from build123d import *

# Parameters (mm, degrees)
SKETCH4_W           = 40
SKETCH4_H           = 85
BOSS_EXTRUDE1_DEPTH = 2.5
SKETCH5_W           = 9.5
SKETCH5_H           = 5
BOSS_EXTRUDE2_DEPTH = 2.5
SKETCH12_W          = 9
SKETCH12_H          = 13
CUT_EXTRUDE1_DEPTH  = 5
FILLET4_R           = 1
FILLET5_R           = 1
SKETCH13_R          = 0.75
CUT_EXTRUDE2_DEPTH  = 10


with BuildPart() as part:
    # Sketch4 → Boss-Extrude1 (new body)
    with BuildSketch(Plane(origin=(0, 0, 0), x_dir=(1, 0, 0), z_dir=(0, 1, 0))):
        Rectangle(SKETCH4_W, SKETCH4_H)
    extrude(amount=BOSS_EXTRUDE1_DEPTH)

    # Sketch5 → Boss-Extrude2 (add)
    with BuildSketch(Plane(origin=(0, 2.5, 0), x_dir=(1, 0, 0), z_dir=(0, 1, 0))):
        with Locations((15.25, -45)):
            Rectangle(SKETCH5_W, SKETCH5_H)
    extrude(amount=-BOSS_EXTRUDE2_DEPTH)

    # Sketch12 → Cut-Extrude1 (cut)
    with BuildSketch(Plane(origin=(0, 2.5, 0), x_dir=(1, 0, 0), z_dir=(0, 1, 0))):
        with Locations((-12.75, 31)):
            Rectangle(SKETCH12_W, SKETCH12_H)
    extrude(amount=-CUT_EXTRUDE1_DEPTH, mode=Mode.SUBTRACT)

    # Fillet4
    fillet4_edges = [part.edges().sort_by_distance(p)[0] for p in [
        (15.25, 2.5, 47.5),
    ]]
    fillet(fillet4_edges, radius=FILLET4_R)

    # Fillet5
    fillet5_edges = [part.edges().sort_by_distance(p)[0] for p in [
        (15.25, 0, 47.5),
    ]]
    fillet(fillet5_edges, radius=FILLET5_R)

    # Sketch13 → Cut-Extrude2 (cut)
    with BuildSketch(Plane.ZY.offset(-10.5)):
        with Locations((46.35, 1.25)):
            Circle(SKETCH13_R)
    extrude(amount=-CUT_EXTRUDE2_DEPTH, mode=Mode.SUBTRACT)


solid = part.part
Could you check a few things on this model? Use its own coordinates, in mm. A direction names the side the tool comes from. Coordinates: 2 decimals unless noted, no trailing zeros. Order: outer loops, then holes, each group sorted by start corner. A loop starts at its lowest first (then second) coordinate and runs counter-clockwise, first axis right, second up.
Q1. Which directions (+Z, -Z, +X, -X, +Y, -Y) give clear straight access to the entire face, cutting with the end or side of a thin tool? Please do faces 1 (the flat face through (-20, 1, 1)), 2 (the flat face through (-13, 1, -37.5)), 3 (the flat face through (-5, 1, 42.5)).
Q2. Will these pins go through, and if not, where does the flat tip stop? pin 1 (0.8 mm diameter, centred on y = 1, z = 46, fed in from -X); pin 2 (0.9 mm diameter, centred on y = 1.25, z = 46.35, fed in from +X); pin 3 (1.2 mm diameter, centred on x = -0.5, y = 1, fed in from +Z).
Q3. Please list where these lines run through material, in increasing order: L1, parallel to Z at x = -14, y = 0.15; L2, parallel to Y at x = 18, z = 46.35; L3, parallel to Z at x = -7, y = 2.
Q4. Thinking about a two-plate mould opening in Z: for faces 4 (the flat face through (0, 1, -42.5)), 5 (the flat face through (-17.25, 1, -31)), 6 (the flat face through (0, 2.5, 1)), 7 (the flat face through (-8.25, 1, -31)), which applies, released by +Z, released by -Z, zero draft, split by the parting line, or undercut?
Q5. Suppose I cut it at A-A on x = -11. Please give me the cut outline in (y, z), and give its area (3 significant figures).
Q6. Suppose I cut it at B-B on x = 1. Please give me the cut outline in (y, z), and give its area (4 significant figures).
Answer:
1. face 1: +Z, -Z, -X, +Y, -Y
1. face 2: +Y, -Y
1. face 3: +Z, -X, +Y, -Y
2. pin 1: stops at x = 10.5
2. pin 2: passes through
2. pin 3: stops at z = 42.5
3. L1: z = -42.5 to -37.5, -24.5 to 42.5
3. L2: y = 0 to 0.5, 2 to 2.5
3. L3: z = -42.5 to 42.5
4. face 4: released by -Z
4. face 5: undercut
4. face 6: zero draft
4. face 7: undercut
5. outline: (0, -42.5) - (2.5, -42.5) - (2.5, -37.5) - (0, -37.5) - close; (0, -24.5) - (2.5, -24.5) - (2.5, 42.5) - (0, 42.5) - close
5. area: 180 mm2
6. outline: (0, -42.5) - (2.5, -42.5) - (2.5, 42.5) - (0, 42.5) - close
6. area: 212.5 mm2
